The drawing under review shows one solid part. Ordinate dimensions are in mm from its lowest x, y, z. A direction names the side the tool comes from. Coordinates: 2 decimals unless noted, no trailing zeros. Order: outer loops, then holes, each group sorted by start corner. A loop starts at its lowest first (then second) coordinate and runs counter-clockwise, first axis right, second up. Notation, with made-up numbers: (6, -20) -> (17, -20) arc R22 cw to (17, 19) -> close; hole circle Ø4 at (74.5, 13.5). An arc over 180 degrees is marked (long way). Use one line per item in the form item = value.
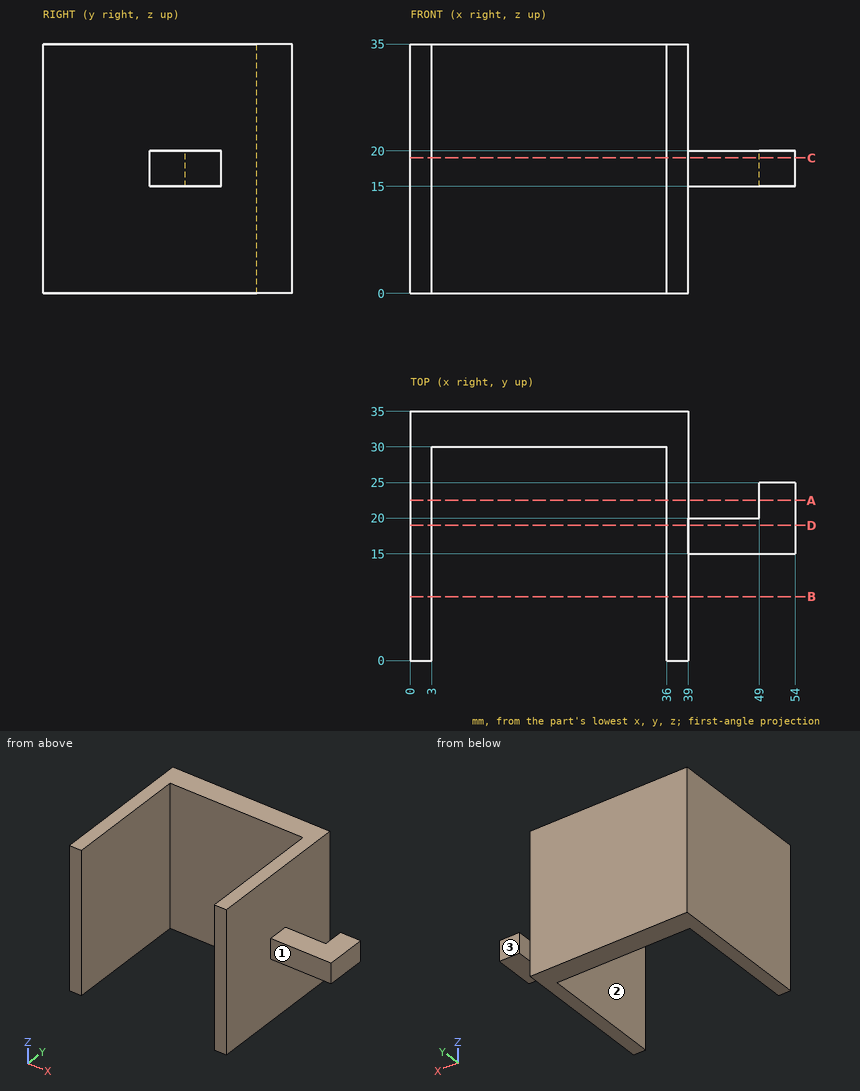
Item 1: Tool access review of the marked faces 1, 2 and 3: name each direction out of +Z, -Z, +X, -X, +Y, -Y from which nothing blocks a thin tool from reaching the whole face with its end or side.
Results found:
face_1 = +Z, -Z, +X, -Y
face_2 = +Z, -Z, -Y
face_3 = +Z, -Z, +X, +Y
Item 2: Clearance check with flat-ended pins moving along their axes: pin 1 (5 mm diameter, centred on x = 19, z = 27, fed in from -Y); pin 2 (1.5 mm diameter, centred on x = 42, z = 17, fed in from +Y); pin 3 (2.5 mm diameter, centred on x = 50.5, z = 17.5, fed in from +Y); pin 4 (5 mm diameter, centred on x = 6.5, y = 9, fed in from -Z). State where each tip first meets the part, or that it passes through.
Results found:
pin_1 = 30
pin_2 = 20
pin_3 = 25
pin_4 = through
Item 3: We need section D-D (y = 19). Write out the cut boundary in (x, z), plus the area to 3 significant figures.
Results found:
outline = (0, 0) -> (3, 0) -> (3, 35) -> (0, 35) -> close; (36, 0) -> (39, 0) -> (39, 15) -> (54, 15) -> (54, 20) -> (39, 20) -> (39, 35) -> (36, 35) -> close
area = 285 mm²
Item 4: We need section B-B (y = 9). Write out the cut boundary in (x, z), plus the area to 3 significant figures.
Results found:
outline = (0, 0) -> (3, 0) -> (3, 35) -> (0, 35) -> close; (36, 0) -> (39, 0) -> (39, 35) -> (36, 35) -> close
area = 210 mm²
Item 5: We need section A-A (y = 22.5). Write out the cut boundary in (x, z).
Results found:
outline = (0, 0) -> (3, 0) -> (3, 35) -> (0, 35) -> close; (36, 0) -> (39, 0) -> (39, 35) -> (36, 35) -> close; (49, 15) -> (54, 15) -> (54, 20) -> (49, 20) -> close
Item 6: To check wall thickness, follow L1, parallel to X at y = 28.5, z = 12; L2, parallel to Y at x = 24.5, z = 14; L3, parallel to Y at x = 49.5, z = 19.5. State the ranges of each line that lie inside material, in increasing order. Write a range as from..to.
Results found:
L1 = 0..3, 36..39
L2 = 30..35
L3 = 15..25
Item 7: We need section C-C (z = 19). Write out the cut boundary in (x, y).
Results found:
outline = (0, 0) -> (3, 0) -> (3, 30) -> (36, 30) -> (36, 0) -> (39, 0) -> (39, 15) -> (54, 15) -> (54, 25) -> (49, 25) -> (49, 20) -> (39, 20) -> (39, 35) -> (0, 35) -> close
